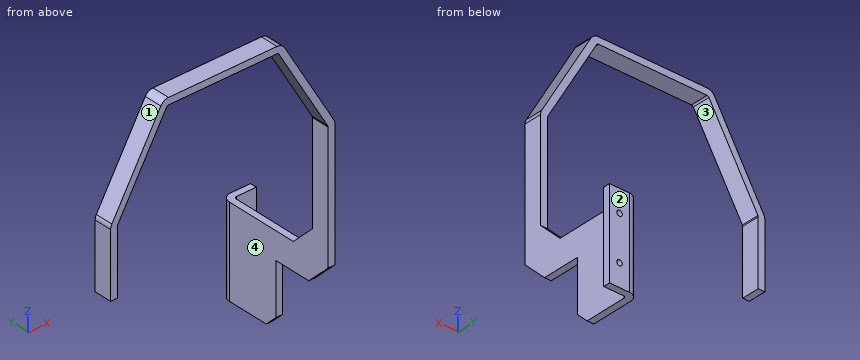
from build123d import *

# Parameters (mm, degrees)
SM_BASE_FLANGE_1_DEPTH           = 40
M3X0_5_1_D                       = 2.5
SKETCH_22_W                      = 3
SKETCH_22_H                      = 12
EXTRUDE_6_DEPTH                  = 19
SKETCH_23_W                      = 3
SKETCH_23_H                      = 67
EXTRUDE_7_DEPTH                  = 8
CHAMFER_1_SIZE                   = 10
CHAMFER_2_SIZE                   = 5
SM_EDGE_FLANGE_1_STRIP_CUT_DEPTH = 8
SM_EDGE_FLANGE_1_DEPTH           = 8
SM_EDGE_FLANGE_2_STRIP_CUT_DEPTH = 8
SM_EDGE_FLANGE_2_DEPTH           = 8
SM_EDGE_FLANGE_3_STRIP_CUT_DEPTH = 8
SM_EDGE_FLANGE_3_DEPTH           = 8
SM_EDGE_FLANGE_4_STRIP_CUT_DEPTH = 8
SM_EDGE_FLANGE_4_DEPTH           = 8


# Sheet-metal steps are written as plain solids
with BuildPart() as part:
    # 草圖3 → 基材-凸緣1 (new body)
    with BuildSketch(Plane.XY):
        with BuildLine():
            Line((10, 0), (1, 0))
            ThreePointArc((1, 0), (0.292893219, -0.292893219), (0, -1))
            Line((0, -1), (0, -25))
            Line((0, -25), (-3, -25))
            Line((-3, -25), (-3, -1))
            ThreePointArc((-3, -1), (-1.828427125, 1.828427125), (1, 3))
            Line((1, 3), (10, 3))
            Line((10, 3), (10, 0))
        make_face()
    extrude(amount=SM_BASE_FLANGE_1_DEPTH)

    # M3x0.5 螺紋孔1 (through all)
    with Locations(Plane(origin=(0, 3, 0), x_dir=(1, 0, 0), z_dir=(0, 1, 0))):
        with Locations((5.5, -30), (5.5, -10)):
            Hole(M3X0_5_1_D / 2)

    # 草圖22 → 填料-伸長6 (add)
    with BuildSketch(Plane.XZ.offset(25)):
        with Locations((-1.5, 34)):
            Rectangle(SKETCH_22_W, SKETCH_22_H)
    extrude(amount=EXTRUDE_6_DEPTH)

    # 草圖23 → 填料-伸長7 (add)
    with BuildSketch(Plane.XZ.offset(44)):
        with Locations((-1.5, 61.5)):
            Rectangle(SKETCH_23_W, SKETCH_23_H)
    extrude(amount=EXTRUDE_7_DEPTH)

    # 導角1
    chamfer_1_edges = [part.edges().sort_by_distance(p)[0] for p in [
        (-1.5, -44, 40),
        (-1.5, -52, 28),
    ]]
    chamfer(chamfer_1_edges, length=CHAMFER_1_SIZE)

    # 導角2
    chamfer_2_edges = [part.edges().sort_by_distance(p)[0] for p in [
        (-1.5, -25, 0),
    ]]
    chamfer(chamfer_2_edges, length=CHAMFER_2_SIZE)

    # 邊線-凸緣1 strip (across the edge) → 邊線-凸緣1 strip cut (cut)
    with BuildSketch(Plane(origin=(-3, -52, 95), x_dir=(-0.8660254037844416, 0, -0.49999999999999495), z_dir=(0, 1, 0))):
        Polygon((-9.464101615, 10.392304845), (-2.464101615, -1.732050808), (0.133974596, -0.232050808), (-6.866025404, 11.892304845), align=None)
    extrude(amount=SM_EDGE_FLANGE_1_STRIP_CUT_DEPTH, mode=Mode.SUBTRACT)

    # 邊線-凸緣1 section (across the edge) → 邊線-凸緣1 (add)
    with BuildSketch(Plane(origin=(-3, -52, 95), x_dir=(-0.8660254037844416, 0, -0.49999999999999495), z_dir=(0, 1, 0))):
        with BuildLine():
            Line((-3, 0.267949192), (-3, 45))
            Line((-3, 45), (0, 45))
            Line((0, 45), (0, 0.267949192))
            ThreePointArc((0, 0.267949192), (0.034074174, 0.009130147), (0.133974596, -0.232050808))
            Line((0.133974596, -0.232050808), (-2.464101615, -1.732050808))
            ThreePointArc((-2.464101615, -1.732050808), (-2.863703305, -0.767326988), (-3, 0.267949192))
        make_face()
    extrude(amount=SM_EDGE_FLANGE_1_DEPTH)

    # 邊線-凸緣2 strip (across the edge) → 邊線-凸緣2 strip cut (cut)
    with BuildSketch(Plane(origin=(-25.5, -52, 133.97114317), x_dir=(0, 0, -1), z_dir=(0, 1, 0))):
        Polygon((-13.124355653, 4.113248654), (-1, -2.886751346), (0.5, -0.288675135), (-11.624355653, 6.711324865), align=None)
    extrude(amount=SM_EDGE_FLANGE_2_STRIP_CUT_DEPTH, mode=Mode.SUBTRACT)

    # 邊線-凸緣2 section (across the edge) → 邊線-凸緣2 (add)
    with BuildSketch(Plane(origin=(-25.5, -52, 133.97114317), x_dir=(0, 0, -1), z_dir=(0, 1, 0))):
        with BuildLine():
            Line((-3, 0.577350269), (-3, 50))
            Line((-3, 50), (0, 50))
            Line((0, 50), (0, 0.577350269))
            ThreePointArc((0, 0.577350269), (0.133974596, 0.077350269), (0.5, -0.288675135))
            Line((0.5, -0.288675135), (-1, -2.886751346))
            ThreePointArc((-1, -2.886751346), (-2.464101615, -1.422649731), (-3, 0.577350269))
        make_face()
    extrude(amount=SM_EDGE_FLANGE_2_DEPTH)

    # 邊線-凸緣3 strip (across the edge) → 邊線-凸緣3 strip cut (cut)
    with BuildSketch(Plane(origin=(-75.5, -52, 133.97114317), x_dir=(0.8660254037844312, -1.5023145987371476e-15, -0.5000000000000132), z_dir=(0, 1, 0))):
        Polygon((-13.124355653, 4.113248654), (-1, -2.886751346), (0.5, -0.288675135), (-11.624355653, 6.711324865), align=None)
    extrude(amount=SM_EDGE_FLANGE_3_STRIP_CUT_DEPTH, mode=Mode.SUBTRACT)

    # 邊線-凸緣3 section (across the edge) → 邊線-凸緣3 (add)
    with BuildSketch(Plane(origin=(-75.5, -52, 133.97114317), x_dir=(0.8660254037844312, -1.5023145987371476e-15, -0.5000000000000132), z_dir=(0, 1, 0))):
        with BuildLine():
            Line((-3, 0.577350269), (-3, 45))
            Line((-3, 45), (0, 45))
            Line((0, 45), (0, 0.577350269))
            ThreePointArc((0, 0.577350269), (0.133974596, 0.077350269), (0.5, -0.288675135))
            Line((0.5, -0.288675135), (-1, -2.886751346))
            ThreePointArc((-1, -2.886751346), (-2.464101615, -1.422649731), (-3, 0.577350269))
        make_face()
    extrude(amount=SM_EDGE_FLANGE_3_DEPTH)

    # 邊線-凸緣4 strip (across the edge) → 邊線-凸緣4 strip cut (cut)
    with BuildSketch(Plane(origin=(-98, -52, 95), x_dir=(1, 0, 0), z_dir=(0, 1, 0))):
        Polygon((-9.464101615, 10.392304845), (-2.464101615, -1.732050808), (0.133974596, -0.232050808), (-6.866025404, 11.892304845), align=None)
    extrude(amount=SM_EDGE_FLANGE_4_STRIP_CUT_DEPTH, mode=Mode.SUBTRACT)

    # 邊線-凸緣4 section (across the edge) → 邊線-凸緣4 (add)
    with BuildSketch(Plane(origin=(-98, -52, 95), x_dir=(1, 0, 0), z_dir=(0, 1, 0))):
        with BuildLine():
            Line((-3, 0.267949192), (-3, 29.196152423))
            Line((-3, 29.196152423), (0, 29.196152423))
            Line((0, 29.196152423), (0, 0.267949192))
            ThreePointArc((0, 0.267949192), (0.034074174, 0.009130147), (0.133974596, -0.232050808))
            Line((0.133974596, -0.232050808), (-2.464101615, -1.732050808))
            ThreePointArc((-2.464101615, -1.732050808), (-2.863703305, -0.767326988), (-3, 0.267949192))
        make_face()
    extrude(amount=SM_EDGE_FLANGE_4_DEPTH)


solid = part.part
Check sheet for the modelled part. Datum: model origin and axes. Units: mm. Face numbers are marked on the shaded views. Round coordinates to 2 decimals unless told otherwise and drop trailing zeros. Loops run counter-clockwise (first coordinate to the right, second up) from the corner with the lowest first, then second, coordinate; pieces in that order, holes last. Notation, with made-up numbers: (7, 22) -> (65, 22) arc R17 cw to (65, 37) -> close; hole circle Ø6 at (4, -3.5). An arc over 180 degrees is marked (long way). Put each result on its own line as item: value. Start each with the question number.
1. Gauge pin test, flat ends, axial feed: pin 1 (0.9 mm diameter, centred on x = -2, y = -30, fed in from -Z); pin 2 (1.5 mm diameter, centred on x = -99, y = -47, fed in from -Z); pin 3 (3 mm diameter, centred on y = -39.5, z = 39.5, fed in from -X); pin 4 (2 mm diameter, centred on x = 5.5, z = 10, fed in from -Y). Record the tip position at first contact, or that the pin passes through.
2. Section check B-B (x = -28). Enter the section's corners in (y, z).
3. Section check A-A (y = -11.5). Enter the section's corners in (x, z), plus the area to 3 significant figures.
4. Scan lines: probe 1 along Z at (x, y) = (5.5, 0.9); probe 2 along Z at (x, y) = (5, 1); probe 3 along X at (y, z) = (-45, 69). Record each from-to range of solid material in increasing order.
5. Draft check along X on the marked faces 1, 2, 3 and 4. Enter one of: +X half, -X half, draft (parallel to the pull), parting line (faces both ways), or undercut.
Findings:
1. pin 1: stops at z = 28
1. pin 2: stops at z = 65.8
1. pin 3: stops at x = -3
1. pin 4: passes through
2. outline: (-52, 133.97) -> (-44, 133.97) -> (-44, 136.97) -> (-52, 136.97) -> close
3. outline: (-3, 0) -> (0, 0) -> (0, 40) -> (-3, 40) -> close
3. area: 120 mm^2
4. probe 1: z = 0 to 8.75, 11.25 to 28.75, 31.25 to 40
4. probe 2: z = 0 to 8.85, 11.15 to 28.85, 31.15 to 40
4. probe 3: x = -101 to -98, -3 to 0
5. face 1: -X half
5. face 2: draft
5. face 3: undercut
5. face 4: undercut
